```python
from build123d import *

# Parameters (mm, degrees)
BOSS_EXTRUDE1_DEPTH = 66
CUT_EXTRUDE1_DEPTH  = 92.290744328
BOSS_EXTRUDE2_START = -6
BOSS_EXTRUDE2_DEPTH = 6
BOSS_EXTRUDE3_DEPTH = 6


with BuildPart() as part:
    # Sketch1 → Boss-Extrude1 (new body)
    with BuildSketch(Plane.YZ):
        with BuildLine():
            Line((0, 0), (0, -15))
            Line((0, -15), (-3, -15))
            Line((-3, -15), (-3, -20))
            Line((-3, -20), (0, -20))
            Line((0, -20), (54, -20))
            Line((54, -20), (57, -20))
            Line((57, -20), (57, -15))
            Line((57, -15), (54, -15))
            Line((54, -15), (54, 0))
            ThreePointArc((54, 0), (27, 27), (0, 0))
        make_face()
    extrude(amount=BOSS_EXTRUDE1_DEPTH)

    # Sketch2 → Cut-Extrude1 (cut, through all)
    with BuildSketch(Plane.YZ.offset(66)):
        with BuildLine():
            Line((6, 0), (6, -20))
            Line((6, -20), (48, -20))
            Line((48, -20), (48, 0))
            ThreePointArc((48, 0), (27, 21), (6, 0))
        make_face()
    extrude(amount=-CUT_EXTRUDE1_DEPTH, mode=Mode.SUBTRACT)

    # Sketch3 → Boss-Extrude2 (add)
    with BuildSketch(Plane.YZ.offset(66).offset(BOSS_EXTRUDE2_START)):
        with BuildLine():
            Line((-3, -15), (0, -15))
            Line((0, -15), (0, 0))
            ThreePointArc((0, 0), (27, 27), (54, 0))
            Line((54, 0), (54, -15))
            Line((54, -15), (57, -15))
            Line((57, -15), (57, 0))
            ThreePointArc((57, 0), (27, 30), (-3, 0))
            Line((-3, 0), (-3, -15))
        make_face()
    extrude(amount=BOSS_EXTRUDE2_DEPTH)

    # Sketch4 → Boss-Extrude3 (add)
    with BuildSketch(Plane(origin=(0, 0, 0), x_dir=(0, -1, 0), z_dir=(-1, 0, 0))):
        with BuildLine():
            Line((-54, -15), (-57, -15))
            Line((-57, -15), (-57, 0))
            ThreePointArc((-57, 0), (-27, 30), (3, 0))
            Line((3, 0), (3, -15))
            Line((3, -15), (0, -15))
            Line((0, -15), (0, 0))
            ThreePointArc((0, 0), (-27, 27), (-54, 0))
            Line((-54, 0), (-54, -15))
        make_face()
    extrude(amount=-BOSS_EXTRUDE3_DEPTH)


solid = part.part
```
Can you work these out from the model? Positions are in its coordinate system, mm. A direction names the side the tool comes from. Coordinates: 2 decimals unless noted, no trailing zeros. Write each loop counter-clockwise with the first axis right and the second up, starting at its lowest first coordinate (ties: lowest second). Pieces come first, ordered by that corner, then holes. Notation, with made-up numbers: M 85.25,34 L 110.25,34 A18 cw 110.25,54 Z; hole C -25.75,64 d4. An arc over 180 degrees is marked long. Answer as CSV lines item,"result".
Item 1: We'd pull the mould along Y, two halves only. Please class faces 1 (the flat face through (33, -3, -17)), 2 (the cylindrical face through (33, 27, 21)), 3 (the flat face through (33, 54, -8)): +Y half, -Y half, draft (parallel to the pull), parting line (faces both ways), or undercut.
Geometry results:
face 1,"-Y half"
face 2,"undercut"
face 3,"+Y half"
Item 2: I'm going to push flat-ended pins straight in: P1, Ø12, axis at x = 24.5, z = -8, coming from the -Y side; P2, Ø4.5, axis at x = 31.5, z = -7.5, coming from the +Y side; P3, Ø1.5, axis at x = 38.5, y = 56, coming from the +Z side. Where does each tip first touch, or does it pass through?
Geometry results:
P1,"stops at y = 0"
P2,"stops at y = 54"
P3,"stops at z = -15"
Item 3: Imagine slicing it at D-D on z = 22. List the corners of the cut face in (x, y) for me.
Geometry results:
outline,"M 0,6.6 L 6,6.6 L 6,11.35 L 60,11.35 L 60,6.6 L 66,6.6 L 66,47.4 L 60,47.4 L 60,42.65 L 6,42.65 L 6,47.4 L 0,47.4 Z"
Item 4: Imagine slicing it at C-C on y = 27. List the corners of the cut face in (x, z) for me, plus the area to 3 significant figures.
Geometry results:
outline,"M 0,21 L 66,21 L 66,30 L 60,30 L 60,27 L 6,27 L 6,30 L 0,30 Z"
area,"432 mm2"
Item 5: Please list where these lines run through material, in increasing order: line 1 along X through (y, z) = (43, 22); line 2 along Y through (x, z) = (34, -2); line 3 along Y through (x, z) = (58, 13).
Geometry results:
line 1,"x = 0 to 6, 60 to 66"
line 2,"y = 0 to 6, 48 to 54"
line 3,"y = 3.34 to 10.51, 43.49 to 50.66"
Item 6: Imagine slicing it at B-B on x = 14. List the corners of the cut face in (y, z) for me.
Geometry results:
outline,"M -3,-20 L 6,-20 L 6,0 A21 cw 48,0 L 48,-20 L 57,-20 L 57,-15 L 54,-15 L 54,0 A27 ccw 0,0 L 0,-15 L -3,-15 Z"
Item 7: Imagine slicing it at A-A on z = -8.5. List the corners of the cut face in (x, y) for me.
Geometry results:
outline,"M 0,-3 L 6,-3 L 6,0 L 60,0 L 60,-3 L 66,-3 L 66,6 L 0,6 Z; M 0,48 L 66,48 L 66,57 L 60,57 L 60,54 L 6,54 L 6,57 L 0,57 Z"
Item 8: On a 3-axis mill with a long thin cutter (end or side, diameter ignored), from which of +Z, -Z, +X, -X, +Y, -Y can I reach the whole of each face in a straight line? I mean faces 4 (the cylindrical face through (32.622, 27.594, 26.993)), 5 (the flat face through (33, -1, -15)), 6 (the flat face through (33, 6, -10)). Say none if no direction works.
Geometry results:
face 4,"+Z"
face 5,"+Z, -Y"
face 6,"-Z, +X, -X"
